Model file for the job. Use its own axes, mm. A direction names the side the tool comes from. Coordinates: 2 decimals unless noted, no trailing zeros. Order: outer loops, then holes, each group sorted by start corner. A loop starts at its lowest first (then second) coordinate and runs counter-clockwise, first axis right, second up. Notation, with made-up numbers: (16, 72.25) - (38, 72.25) arc R15 ccw to (38, 79.25) - close; hole circle Ø5 at (56, 64). An arc over 180 degrees is marked (long way). Put each result on its own line as item: value. Start each with the question number.
```python
from build123d import *

# Parameters (mm, degrees)
SKETCH_1_R      = 1.102856911
EXTRUDE_1_DEPTH = 182


with BuildPart() as part:
    # 草图1 → 凸台-拉伸1 (new body)
    with BuildSketch(Plane.XY):
        with BuildLine():
            Line((1, 45), (3, 45))
            Line((3, 45), (3, 43))
            Line((3, 43), (10, 43))
            Line((10, 43), (10, 41.324203171))
            Line((10, 41.324203171), (7.873486532, 37.954843198))
            Line((7.873486532, 37.954843198), (4.832988285, 37.954843198))
            Line((4.832988285, 37.954843198), (3, 40))
            Line((3, 40), (3, 5))
            Line((3, 5), (4.832988285, 7.045156802))
            Line((4.832988285, 7.045156802), (7.873486532, 7.045156802))
            Line((7.873486532, 7.045156802), (10, 3.675796829))
            Line((10, 3.675796829), (10, 2))
            Line((10, 2), (3, 2))
            Line((3, 2), (3, 0))
            Line((3, 0), (1, 0))
            ThreePointArc((1, 0), (0.292893219, 0.292893219), (0, 1))
            Line((0, 1), (0, 44))
            ThreePointArc((0, 44), (0.292893219, 44.707106781), (1, 45))
        make_face()
        with Locations((6.5, 5)):
            Circle(SKETCH_1_R, mode=Mode.SUBTRACT)
        with Locations((6.5, 40)):
            Circle(SKETCH_1_R, mode=Mode.SUBTRACT)
    extrude(amount=EXTRUDE_1_DEPTH)


solid = part.part
```
Item 1: 3-axis set-ups, long thin cutter, end or side, ignore diameter. For faces 1 (the face through (7, 2, 90)), 2 (the face through (2.8, 22.8, 0)), 3 (the face through (8.95, 39.66, 89.73)): which of +Z, -Z, +X, -X, +Y, -Y reach the whole face in a straight line?
Item 2: Pull direction Y, two halves, no side cores. Call faces 4 (the face through (6, 43, 90)), 5 (the face through (2.8, 22.8, 182)), 6 (the face through (6, 37.955, 90)): pulls with the +Y half, pulls with the -Y half, needs draft (parallel to the pull), parting line crosses it, or undercut.
Item 3: Slice it at A-A, the plane z = 23. Give the cut face in (x, y), plus the area to 3 significant figures.
Item 4: Wall check: line 1 along Y through (x, z) = (6.5, 118); line 2 along Y through (x, z) = (3.5, 77.5); line 3 along X through (y, z) = (5.5, 149.5). Give the ranges that are in metal, low to high.
Item 5: Slice it at B-B, the plane y = 16.5. Give the cut face in (x, z).
Item 6: Flat gauge pins, fed straight in: pin 1 Ø3 at (x, z) = (7, 163.5) entering from +Y; pin 2 Ø0.6 at (y, z) = (43.5, 95) entering from +X; pin 3 Ø1.5 at (x, z) = (6.5, 97.5) entering from -Y. Where does each tip first touch, or does it go through?
Here are the results:
1. face 1: +Z, -Z, +X, -Y
1. face 2: -Z, +X, -X, +Y, -Y
1. face 3: +Z, -Z, +X
2. face 4: pulls with the +Y half
2. face 5: needs draft
2. face 6: undercut
3. outline: (0, 1) arc R1 ccw to (1, 0) - (3, 0) - (3, 2) - (10, 2) - (10, 3.68) - (7.87, 7.05) - (4.83, 7.05) - (3, 5) - (3, 40) - (4.83, 37.95) - (7.87, 37.95) - (10, 41.32) - (10, 43) - (3, 43) - (3, 45) - (1, 45) arc R1 ccw to (0, 44) - close; hole circle Ø2.21 at (6.5, 5); hole circle Ø2.21 at (6.5, 40)
3. area: 187 mm^2
4. line 1: y = 2 to 3.9, 6.1 to 7.05, 37.95 to 38.9, 41.1 to 43
4. line 2: y = 2 to 5.56, 39.44 to 43
4. line 3: x = 0 to 3, 3.45 to 5.52, 7.48 to 8.85
5. outline: (0, 0) - (3, 0) - (3, 182) - (0, 182) - close
6. pin 1: stops at y = 43
6. pin 2: stops at x = 3
6. pin 3: stops at y = 2
